from build123d import *

# Parameters (mm, degrees)
F0_R     = 6.35
F1_DEPTH = 1
F2_W     = 180
F2_H     = 20
F2_R     = 6.35
F3_DEPTH = 0.2


with BuildPart() as f1:
    # F0 (on Front) → F1 (new body)
    with BuildSketch(Plane.XZ):
        with BuildLine():
            Line((77.3, 78.003146), (-77.3, 78.003146))
            ThreePointArc((-77.3, 78.003146), (-86.280256, 74.283402), (-90, 65.303146))
            Line((-90, 65.303146), (-90, -26.096854))
            Line((-90, -26.096854), (90, -26.096854))
            Line((90, -26.096854), (90, 65.303146))
            ThreePointArc((90, 65.303146), (86.280256, 74.283402), (77.3, 78.003146))
        make_face()
        with Locations((-68.2625, -14.846854)):
            Circle(F0_R, mode=Mode.SUBTRACT)
        with Locations((68.2625, -14.846854)):
            Circle(F0_R, mode=Mode.SUBTRACT)
        with Locations((-68.2625, 66.753146)):
            Circle(F0_R, mode=Mode.SUBTRACT)
        with Locations((68.2625, 66.753146)):
            Circle(F0_R, mode=Mode.SUBTRACT)
    extrude(amount=F1_DEPTH)

    # F2 (on face) → F3 (join)
    with BuildSketch(Plane.XZ.offset(1)):
        with Locations((0, -16.096854)):
            Rectangle(F2_W, F2_H)
        with Locations((-68.2625, -14.846854)):
            Circle(F2_R, mode=Mode.SUBTRACT)
        with Locations((68.2625, -14.846854)):
            Circle(F2_R, mode=Mode.SUBTRACT)
    extrude(amount=F3_DEPTH)


solid = f1.part
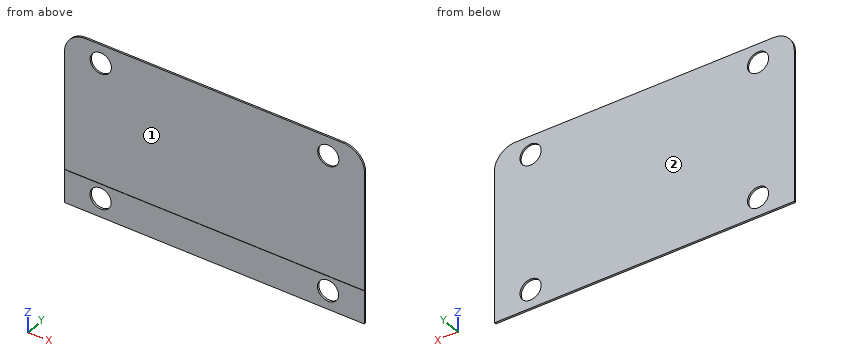
Source: CAD feature listing. Evaluate the final solid. Frame: model axes, mm. Face numbers are marked on the shaded views. A direction names the side the tool comes from. Give positions to 0.01 mm unless a question says otherwise; leave off trailing zeros. Write each loop counter-clockwise with the first axis right and the second up, starting at its lowest first coordinate (ties: lowest second). Pieces come first, ordered by that corner, then holes. Notation, with made-up numbers: (66.25, -31) - (83.25, -31) arc R14 ccw to (83.25, -9) - close; hole circle Ø3 at (4.5, 7.25). An arc over 180 degrees is marked (long way). Write item = value, one per line. Start each with the question number.
Q1. Cut plane D-D, the plane x = 46. Return loops of the section in (y, z), then the cut area to 3 significant figures.
Q2. Reachability of the marked faces 1 and 2 from +Z, -Z, +X, -X, +Y, -Y: full face, straight path, thin tool, end or side. Return the list, or none.
Q3. Cut plane B-B, the plane x = -72.5. Return loops of the section in (y, z).
Q4. Cut plane C-C, the plane y = -0.35. Return loops of the section in (x, z).
Q5. Pin query (flat end, axial travel): pin 1 Ø10 at (x, z) = (-68.26, 66.75) entering from -Y; pin 2 Ø4 at (x, z) = (23.5, 43.5) entering from -Y. Return the tip coordinate at first contact, or that it passes through.
Q6. Material intervals for probe 1 along X at (y, z) = (-0.3, -12); probe 2 along Z at (x, y) = (-69, -0.2); probe 3 along X at (y, z) = (-0.8, 61), sorted ascending.
Q7. Cut plane A-A, the plane z = -13. Return loops of the section in (x, y), then the cut area to 3 significant figures.
Computed values:
q1.outline = (-1.2, -26.1) - (0, -26.1) - (0, 78) - (-1, 78) - (-1, -6.1) - (-1.2, -6.1) - close
q1.area = 108 mm²
q2.face_1 = +Z, +X, -X, -Y
q2.face_2 = +Z, -Z, +X, -X, +Y
q3.outline = (-1.2, -26.1) - (0, -26.1) - (0, -19.58) - (-1.2, -19.58) - close; (-1.2, -10.12) - (0, -10.12) - (0, 62.02) - (-1, 62.02) - (-1, -6.1) - (-1.2, -6.1) - close; (-1, 71.48) - (0, 71.48) - (0, 78) - (-1, 78) - close
q4.outline = (-90, -26.1) - (90, -26.1) - (90, 65.3) arc R12.7 ccw to (77.3, 78) - (-77.3, 78) arc R12.7 ccw to (-90, 65.3) - close; hole circle Ø12.7 at (-68.26, -14.85); hole circle Ø12.7 at (-68.26, 66.75); hole circle Ø12.7 at (68.26, -14.85); hole circle Ø12.7 at (68.26, 66.75)
q5.pin_1 = through
q5.pin_2 = -1
q6.probe_1 = -90 to -73.94, -62.59 to 62.59, 73.94 to 90
q6.probe_2 = -26.1 to -21.15, -8.54 to 60.45, 73.06 to 78
q6.probe_3 = -90 to -70.95, -65.57 to 65.57, 70.95 to 90
q7.outline = (-90, -1.2) - (-74.34, -1.2) - (-74.34, 0) - (-90, 0) - close; (-62.19, -1.2) - (62.19, -1.2) - (62.19, 0) - (-62.19, 0) - close; (74.34, -1.2) - (90, -1.2) - (90, 0) - (74.34, 0) - close
q7.area = 187 mm²
